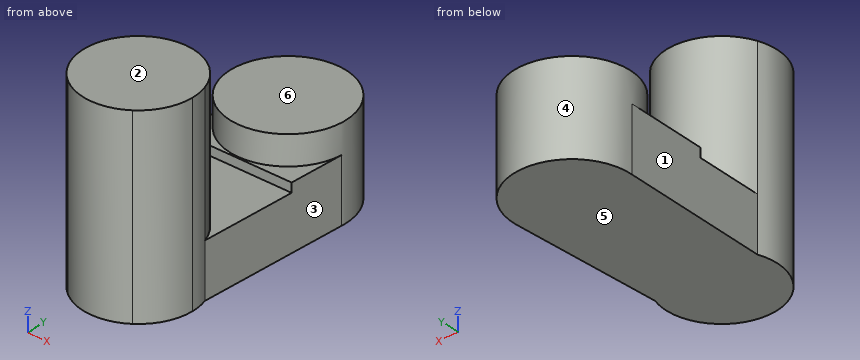
from build123d import *

# Parameters (mm, degrees)
F1_DEPTH = 368.3
F0_W     = 105.1427514449
F0_H     = 53.7366458577
F2_DEPTH = 104.14
F3_DEPTH = 121.92
F4_DEPTH = 177.8


with BuildPart() as f1:
    # F0 (on Top) → F1 (new body)
    with BuildSketch(Plane.XY):
        Polygon((0, -167.1104878187), (-63.1326169969, -252.2933322156), (63.1326169969, -252.2933322156), align=None)
        with BuildLine():
            ThreePointArc((106.0275639087, -167.1104878187), (104.5706585234, -149.5941615946), (100.2399805091, -132.5592126476))
            Line((100.2399805091, -132.5592126476), (0, -132.5592126476))
            Line((0, -132.5592126476), (0, -167.1104878187))
            Line((0, -167.1104878187), (63.1326169969, -252.2933322156))
            ThreePointArc((63.1326169969, -252.2933322156), (94.6985794291, -214.797208848), (106.0275639087, -167.1104878187))
        make_face()
        with BuildLine():
            Line((0, -132.5592126476), (-100.2399805091, -132.5592126476))
            ThreePointArc((-100.2399805091, -132.5592126476), (-101.275447425, -198.4972375273), (-63.1326169969, -252.2933322156))
            Line((-63.1326169969, -252.2933322156), (0, -167.1104878187))
            Line((0, -167.1104878187), (0, -132.5592126476))
        make_face()
        Polygon((0, -61.08292391), (-100.2399805091, -132.5592126476), (0, -132.5592126476), align=None)
        Polygon((0, -132.5592126476), (100.2399805091, -132.5592126476), (0, -61.08292391), align=None)
        with BuildLine():
            Line((63.1326169969, -252.2933322156), (-63.1326169969, -252.2933322156))
            ThreePointArc((-63.1326169969, -252.2933322156), (0, -273.1380517274), (63.1326169969, -252.2933322156))
        make_face()
        with BuildLine():
            ThreePointArc((0, -61.08292391), (-61.5567087005, -80.7819530091), (-100.2399805091, -132.5592126476))
            Line((-100.2399805091, -132.5592126476), (0, -61.08292391))
        make_face()
        with BuildLine():
            Line((0, -61.08292391), (100.2399805091, -132.5592126476))
            ThreePointArc((100.2399805091, -132.5592126476), (61.5567087005, -80.7819530091), (0, -61.08292391))
        make_face()
    extrude(amount=F1_DEPTH)

    # F0 (on Top) → F2 (join)
    with BuildSketch(Plane.XY):
        with BuildLine():
            Line((0, 0), (-105.1427514449, 0))
            Line((-105.1427514449, 0), (-100.2399805091, -132.5592126476))
            ThreePointArc((-100.2399805091, -132.5592126476), (-61.5567087005, -80.7819530091), (0, -61.08292391))
            Line((0, -61.08292391), (0, 0))
        make_face()
        with BuildLine():
            Line((100.2399805091, -132.5592126476), (105.1427514449, 0))
            Line((105.1427514449, 0), (0, 0))
            Line((0, 0), (0, -61.08292391))
            ThreePointArc((0, -61.08292391), (61.5567087005, -80.7819530091), (100.2399805091, -132.5592126476))
        make_face()
        Polygon((105.1427514449, 0), (107.1302290426, 53.7366458577), (0, 53.7366458577), (0, 0), align=None)
        with Locations((-52.5713757225, 26.8683229289)):
            Rectangle(F0_W, F0_H)
    extrude(amount=F2_DEPTH)

    # F0 (on Top) → F3 (join)
    with BuildSketch(Plane.XY):
        with BuildLine():
            Line((0, 53.7366458577), (0, 56.7909614803))
            ThreePointArc((0, 56.7909614803), (-76.0917297258, 86.8530505453), (-111.0901819179, 160.8043106819))
            Line((-111.0901819179, 160.8043106819), (-105.1427514449, 0))
            Line((-105.1427514449, 0), (-105.1427514449, 53.7366458577))
            Line((-105.1427514449, 53.7366458577), (0, 53.7366458577))
        make_face()
        with BuildLine():
            Line((107.1302290426, 53.7366458577), (111.0901819179, 160.8043106819))
            ThreePointArc((111.0901819179, 160.8043106819), (76.0917297258, 86.8530505453), (0, 56.7909614803))
            Line((0, 56.7909614803), (0, 53.7366458577))
            Line((0, 53.7366458577), (107.1302290426, 53.7366458577))
        make_face()
    extrude(amount=F3_DEPTH)

    # F0 (on Top) → F4 (join)
    with BuildSketch(Plane.XY):
        with BuildLine():
            ThreePointArc((0, 56.7909614803), (76.0917297258, 86.8530505453), (111.0901819179, 160.8043106819))
            Line((111.0901819179, 160.8043106819), (0, 56.7909614803))
        make_face()
        Polygon((0, 56.7909614803), (111.0901819179, 160.8043106819), (0, 160.8043106819), align=None)
        with BuildLine():
            ThreePointArc((-111.0901819179, 160.8043106819), (-76.0917297258, 86.8530505453), (0, 56.7909614803))
            Line((0, 56.7909614803), (-111.0901819179, 160.8043106819))
        make_face()
        with BuildLine():
            Line((0, 168.1218892336), (-63.1326169969, 259.8216610192))
            ThreePointArc((-63.1326169969, 259.8216610192), (-100.1973294673, 216.6509593053), (-111.0901819179, 160.8043106819))
            Line((-111.0901819179, 160.8043106819), (0, 160.8043106819))
            Line((0, 160.8043106819), (0, 168.1218892336))
        make_face()
        Polygon((-111.0901819179, 160.8043106819), (0, 56.7909614803), (0, 160.8043106819), align=None)
        with BuildLine():
            Line((-63.1326169969, 259.8216610192), (63.1326169969, 259.8216610192))
            ThreePointArc((63.1326169969, 259.8216610192), (0, 279.4528169869), (-63.1326169969, 259.8216610192))
        make_face()
        with BuildLine():
            ThreePointArc((111.0901819179, 160.8043106819), (111.270725017, 164.4611203793), (111.3309277533, 168.1218892336))
            ThreePointArc((111.3309277533, 168.1218892336), (98.5474208089, 219.9193923233), (63.1326169969, 259.8216610192))
            Line((63.1326169969, 259.8216610192), (0, 168.1218892336))
            Line((0, 168.1218892336), (0, 160.8043106819))
            Line((0, 160.8043106819), (111.0901819179, 160.8043106819))
        make_face()
        Polygon((0, 168.1218892336), (63.1326169969, 259.8216610192), (-63.1326169969, 259.8216610192), align=None)
    extrude(amount=F4_DEPTH)


solid = f1.part
Input: part model. Units: mm. Frame: model coordinates. Face numbers are marked on the shaded views. A direction names the side the tool comes from. Coordinates: 2 decimals unless noted, no trailing zeros. Loops run counter-clockwise (first coordinate to the right, second up) from the corner with the lowest first, then second, coordinate; pieces in that order, holes last.
Q1. Set-up query: the marked faces 4, 5 and 6. Return all of +Z, -Z, +X, -X, +Y, -Y with unobstructed straight access to the full face (end or side cutting, diameter ignored); none if empty.
Q2. Cut plane C-C (y = 99). Output: boundary loops of the cut face in (x, z).
Q3. Draft query along Y for the marked faces 1, 2 and 3. Return one class per face: +Y half, -Y half, draft (parallel to the pull), parting line (faces both ways), or undercut.
Q4. Cut plane B-B (z = 38.5). Output: boundary loops of the cut face in (x, y), then the cut area to 3 significant figures.
Q5. Contact query for flat-ended pins moving along their axis: pin 1 (6 mm diameter, centred on y = 120.5, z = 79.5, fed in from +X); pin 2 (9 mm diameter, centred on x = -28.5, z = 115, fed in from -Y); pin 3 (1.5 mm diameter, centred on x = 46, z = 207.5, fed in from -Y). Output: stop coordinate, or through.
Q6. Material intervals for line 1 (Z direction, x = 66, y = 76); line 2 (Z direction, x = 81, y = 220); line 3 (Y direction, x = -59.5, z = 155.5), sorted ascending.
Q7. Cut plane D-D (x = -48). Output: boundary loops of the cut face in (y, z), then the cut area to 3 significant figures.
Q8. Cut plane A-A (x = 0). Output: boundary loops of the cut face in (y, z).
Working result:
1. face 4: +Z
1. face 5: -Z, +X, -X, +Y, -Y
1. face 6: +Z, +X, -X, +Y
2. outline: (-108.8, 0) - (108.8, 0) - (108.8, 121.92) - (87.27, 121.92) - (87.27, 177.8) - (-87.27, 177.8) - (-87.27, 121.92) - (-108.8, 121.92) - close
3. face 1: undercut
3. face 2: draft
3. face 3: undercut
4. outline: (-111.09, 160.8) - (-100.24, -132.56) arc R106.03 ccw (long way) to (100.24, -132.56) - (111.09, 160.8) arc R111.33 ccw (long way) to start
4. area: 108,000 mm2
5. pin 1: stops at x = 109.71
5. pin 2: stops at y = -270.39
5. pin 3: stops at y = -263
6. line 1: z = 0 to 121.92
6. line 2: z = 0 to 177.8
6. line 3: y = -254.87 to -79.35, 74.02 to 262.22
7. outline: (-261.65, 0) - (268.57, 0) - (268.57, 177.8) - (67.67, 177.8) - (67.67, 121.92) - (53.74, 121.92) - (53.74, 104.14) - (-72.57, 104.14) - (-72.57, 368.3) - (-261.65, 368.3) - close
7. area: 120,000 mm2
8. outline: (-273.14, 0) - (279.45, 0) - (279.45, 177.8) - (56.79, 177.8) - (56.79, 121.92) - (53.74, 121.92) - (53.74, 104.14) - (-61.08, 104.14) - (-61.08, 368.3) - (-273.14, 368.3) - close
